```python
from build123d import *

# Parameters (mm, degrees)
CUT_EXTRUDE1_DEPTH = 2.5


with BuildPart() as part:
    # Sketch1 → Revolve1 (revolve)
    with BuildSketch(Plane.XY, mode=Mode.PRIVATE) as revolve1_sk:
        Polygon((4, 4.5), (0, 4.5), (0, 0), (20, 0), (20, 2), (12, 2), (12, 2.5), (4, 2.5), align=None)
    revolve(revolve1_sk.sketch.rotate(Axis((-20, 0, 0), (1, 0, 0)), 90), axis=Axis((-20, 0, 0), (1, 0, 0)))

    # Sketch2 → Cut-Extrude1 (cut)
    with BuildSketch(Plane.ZY):
        Polygon((1.443375673, 0), (0.721687836, 1.25), (-0.721687836, 1.25), (-1.443375673, 0), (-0.721687836, -1.25), (0.721687836, -1.25), align=None)
    extrude(amount=-CUT_EXTRUDE1_DEPTH, mode=Mode.SUBTRACT)


solid = part.part
```
For this review, take the finished solid that the model builds, in its own axes (mm). A direction names the side the tool comes from. Coordinates: 2 decimals unless noted, no trailing zeros. Write each loop counter-clockwise with the first axis right and the second up, starting at its lowest first coordinate (ties: lowest second). Pieces come first, ordered by that corner, then holes. Notation, with made-up numbers: (-26, -36) -> (17, -36) arc R22 cw to (17, -6) -> close; hole circle Ø1 at (4.5, 2). An arc over 180 degrees is marked (long way). Put each result on its own line as item: value.
Q1. Wall thickness on L1, parallel to X at y = 1.5, z = 3.25; L2, parallel to Z at x = 10.5, y = -1.5: over which ranges is each line inside the solid? List them lowest first.
From the geometry:
L1: x = 0 to 4
L2: z = -2 to 2
Q2. The part is to be moulded in two halves that separate along Z. For faces 1 (the flat face through (12, -2, 1)), 2 (the cylindrical face through (1.97, -3.04, -3.32)), 3 (the flat face through (1.232, -0.616, -1.088)), say which applies: +Z half, -Z half, draft (parallel to the pull), parting line (faces both ways), or undercut.
From the geometry:
face 1: draft
face 2: parting line
face 3: undercut
Q3. Tool access review of faces 4 (the flat face through (1.23, -0.63, 1.08)), 5 (the flat face through (20, 0, 0)), 6 (the cylindrical face through (7.9, -0.1, -2.5)): name each direction out of +Z, -Z, +X, -X, +Y, -Y from which nothing blocks a thin tool from reaching the whole face with its end or side.
From the geometry:
face 4: -X
face 5: +Z, -Z, +X, +Y, -Y
face 6: +X
Q4. Take a section at A-A, the plane z = 0. State the section outline as (x, y) points.
From the geometry:
outline: (0, -4.5) -> (4, -4.5) -> (4, -2.5) -> (12, -2.5) -> (12, -2) -> (20, -2) -> (20, 2) -> (12, 2) -> (12, 2.5) -> (4, 2.5) -> (4, 4.5) -> (0, 4.5) -> (0, 1.25) -> (2.5, 1.25) -> (2.5, -1.25) -> (0, -1.25) -> close
Q5. Clearance check with flat-ended pins moving along their axes: pin 1 Ø1.5 at (x, z) = (9.5, 3) entering from +Y; pin 2 Ø0.8 at (y, z) = (-0.5, 0.5) entering from -X; pin 3 Ø1.5 at (x, z) = (10, 0) entering from +Y. State where each tip first meets the part, or that it passes through.
From the geometry:
pin 1: stops at y = 1.09
pin 2: stops at x = 2.5
pin 3: stops at y = 2.5
Q6. Take a section at B-B, the plane y = 0.5. State the section outline as (x, z) points, then the cut area to 3 significant figures.
From the geometry:
outline: (0, -4.47) -> (4, -4.47) -> (4, -2.45) -> (12, -2.45) -> (12, -1.94) -> (20, -1.94) -> (20, 1.94) -> (12, 1.94) -> (12, 2.45) -> (4, 2.45) -> (4, 4.47) -> (0, 4.47) -> (0, 1.15) -> (2.5, 1.15) -> (2.5, -1.15) -> (0, -1.15) -> close
area: 100 mm2
Q7. Take a section at C-C, the plane x = 17.5. State the section outline as (y, z) points.
From the geometry:
outline: circle Ø4 at (0, 0)
Q8. Take a section at D-D, the plane z = 2.25. State the section outline as (x, y) points.
From the geometry:
outline: (0, -3.9) -> (4, -3.9) -> (4, -1.09) -> (12, -1.09) -> (12, 1.09) -> (4, 1.09) -> (4, 3.9) -> (0, 3.9) -> close
